from build123d import *

# Parameters (mm, degrees)
F1_DEPTH = 240
F0_W     = 160
F0_H     = 48
F0_W_2   = 40
F0_W_3   = 152
F0_H_2   = 202
F0_W_4   = 50
F0_H_3   = 150
F0_H_4   = 50
F2_DEPTH = 3
F3_DEPTH = 201
F4_DEPTH = 55
F5_DEPTH = 60
F6_DEPTH = 78


with BuildPart() as f1:
    # F0 (on Top) → F1 (new body)
    with BuildSketch(Plane.XY):
        Polygon((145, -391.5), (145, -373), (208, -373), (208, -391.5), (399.5, -391.5), (399.5, -68.5), (91, -68.5), (91, 10), (-10, 10), (-10, -391.5), align=None)
        Polygon((0, -381.5), (0, 0), (81, 0), (81, -78.5), (389.5, -78.5), (389.5, -381.5), (218, -381.5), (218, -363), (135, -363), (135, -381.5), align=None, mode=Mode.SUBTRACT)
    extrude(amount=F1_DEPTH)

    # F0 (on Top) → F2 (join)
    with BuildSketch(Plane.XY):
        Polygon((145, -391.5), (145, -373), (208, -373), (208, -391.5), (399.5, -391.5), (399.5, -68.5), (91, -68.5), (91, 10), (-10, 10), (-10, -391.5), align=None)
        Polygon((0, -381.5), (0, 0), (81, 0), (81, -78.5), (389.5, -78.5), (389.5, -381.5), (218, -381.5), (218, -363), (135, -363), (135, -381.5), align=None, mode=Mode.SUBTRACT)
        Polygon((81, 0), (0, 0), (0, -381.5), (135, -381.5), (135, -363), (218, -363), (218, -381.5), (389.5, -381.5), (389.5, -78.5), (81, -78.5), align=None)
        Polygon((2, -306.5), (2, -156.5), (52, -156.5), (52, -306.5), (75, -329.5), (125, -329.5), (125, -379.5), (75, -379.5), (2, -379.5), align=None, mode=Mode.SUBTRACT)
        with Locations((304.5, -355.5)):
            Rectangle(F0_W, F0_H, mode=Mode.SUBTRACT)
        with Locations((123.5, -107.5)):
            Rectangle(F0_W_2, F0_H, mode=Mode.SUBTRACT)
        with Locations((224.5, -184.5)):
            Rectangle(F0_W_3, F0_H_2, mode=Mode.SUBTRACT)
        with Locations((325.5, -107.5)):
            Rectangle(F0_W_2, F0_H, mode=Mode.SUBTRACT)
        with Locations((27, -231.5)):
            Rectangle(F0_W_4, F0_H_3)
        with Locations((224.5, -184.5)):
            Rectangle(F0_W_3, F0_H_2)
        with Locations((123.5, -107.5)):
            Rectangle(F0_W_2, F0_H)
        with Locations((325.5, -107.5)):
            Rectangle(F0_W_2, F0_H)
        with Locations((304.5, -355.5)):
            Rectangle(F0_W, F0_H)
        Polygon((52, -306.5), (2, -306.5), (2, -379.5), (75, -379.5), (75, -329.5), align=None)
        with Locations((100, -354.5)):
            Rectangle(F0_W_4, F0_H_4)
    extrude(amount=-F2_DEPTH)

    # F0 (on Top) → F3 (join)
    with BuildSketch(Plane.XY):
        with Locations((27, -231.5)):
            Rectangle(F0_W_4, F0_H_3)
        Polygon((52, -306.5), (2, -306.5), (2, -379.5), (75, -379.5), (75, -329.5), align=None)
        with Locations((100, -354.5)):
            Rectangle(F0_W_4, F0_H_4)
    extrude(amount=F3_DEPTH)

    # F0 (on Top) → F4 (join)
    with BuildSketch(Plane.XY):
        with Locations((123.5, -107.5)):
            Rectangle(F0_W_2, F0_H)
        with Locations((325.5, -107.5)):
            Rectangle(F0_W_2, F0_H)
    extrude(amount=F4_DEPTH)

    # F0 (on Top) → F5 (join)
    with BuildSketch(Plane.XY):
        with Locations((224.5, -184.5)):
            Rectangle(F0_W_3, F0_H_2)
    extrude(amount=F5_DEPTH)

    # F0 (on Top) → F6 (join)
    with BuildSketch(Plane.XY):
        with Locations((304.5, -355.5)):
            Rectangle(F0_W, F0_H)
    extrude(amount=F6_DEPTH)


solid = f1.part
The model under review builds one solid part; all positions refer to its coordinate system, in mm. A direction names the side the tool comes from. Give positions to 0.01 mm unless a question says otherwise; leave off trailing zeros. Order: outer loops, then holes, each group sorted by start corner. A loop starts at its lowest first (then second) coordinate and runs counter-clockwise, first axis right, second up. Notation, with made-up numbers: (69.25, 30) -> (105.25, 30) arc R16 ccw to (105.25, 45) -> close; hole circle Ø10 at (78, 8). An arc over 180 degrees is marked (long way). Write item = value, one per line. Start each with the question number.
(1) For pin 1 Ø20 at (x, y) = (132, -114.5) entering from +Z; pin 2 Ø12 at (x, y) = (37, -60.5) entering from +Z; pin 3 Ø1.5 at (x, y) = (48, -185.5) entering from +Z, all flat-tipped, find the tip position at first contact; note any pin that passes through.
(2) Take a section at A-A (z = 146). Write out the cut boundary in (x, y).
(3) Tool access review of faces 5 (the flat face through (52, -233, 99)), 6 (the flat face through (247, -68.5, 120)), 7 (the flat face through (176, -373, 120)): name each direction out of +Z, -Z, +X, -X, +Y, -Y from which nothing blocks a thin tool from reaching the whole face with its end or side.
(4) Take a section at C-C (y = -226). Write out the cut boundary in (x, z).
(5) Take a section at D-D (x = 157). Write out the cut boundary in (y, z), plus the area to 3 significant figures.
(6) Take a section at B-B (z = 224.5). Write out the cut boundary in (x, y).
(7) For L1, parallel to Y at x = 333, z = 54; L2, parallel to Y at x = 281.5, z = 38; L3, parallel to X at y = -365, z = 199, list the stretches that pass through material, from the lowest coordinate up. Write a range as from..to.
(8) Draft analysis for pull direction X (two halves, no side actions). For faces 1 (the flat face through (223, -83.5, 30)), 2 (the flat face through (302, -391.5, 120)), 3 (the flat face through (0, -193, 118)), 4 (the flat face through (399.5, -232, 120)), state which applies: +X half, -X half, draft (parallel to the pull), parting line (faces both ways), or undercut.
Returned:
q1.pin_1 = 55
q1.pin_2 = 0
q1.pin_3 = 201
q2.outline = (-10, -391.5) -> (145, -391.5) -> (145, -373) -> (208, -373) -> (208, -391.5) -> (399.5, -391.5) -> (399.5, -68.5) -> (91, -68.5) -> (91, 10) -> (-10, 10) -> close; (2, -379.5) -> (125, -379.5) -> (125, -329.5) -> (75, -329.5) -> (52, -306.5) -> (52, -156.5) -> (2, -156.5) -> close; hole (0, -381.5) -> (135, -381.5) -> (135, -363) -> (218, -363) -> (218, -381.5) -> (389.5, -381.5) -> (389.5, -78.5) -> (81, -78.5) -> (81, 0) -> (0, 0) -> close
q3.face_5 = +Z
q3.face_6 = +Z, -Z, +X, +Y
q3.face_7 = +Z, -Z, -Y
q4.outline = (-10, -3) -> (399.5, -3) -> (399.5, 240) -> (389.5, 240) -> (389.5, 0) -> (300.5, 0) -> (300.5, 60) -> (148.5, 60) -> (148.5, 0) -> (52, 0) -> (52, 201) -> (2, 201) -> (2, 0) -> (0, 0) -> (0, 240) -> (-10, 240) -> close
q5.outline = (-373, -3) -> (-68.5, -3) -> (-68.5, 240) -> (-78.5, 240) -> (-78.5, 0) -> (-83.5, 0) -> (-83.5, 60) -> (-285.5, 60) -> (-285.5, 0) -> (-363, 0) -> (-363, 240) -> (-373, 240) -> close
q5.area = 17,800 mm²
q6.outline = (-10, -391.5) -> (145, -391.5) -> (145, -373) -> (208, -373) -> (208, -391.5) -> (399.5, -391.5) -> (399.5, -68.5) -> (91, -68.5) -> (91, 10) -> (-10, 10) -> close; hole (0, -381.5) -> (135, -381.5) -> (135, -363) -> (218, -363) -> (218, -381.5) -> (389.5, -381.5) -> (389.5, -78.5) -> (81, -78.5) -> (81, 0) -> (0, 0) -> close
q7.L1 = -391.5..-381.5, -379.5..-331.5, -131.5..-83.5, -78.5..-68.5
q7.L2 = -391.5..-381.5, -379.5..-331.5, -285.5..-83.5, -78.5..-68.5
q7.L3 = -10..0, 2..125, 135..218, 389.5..399.5
q8.face_1 = undercut
q8.face_2 = draft
q8.face_3 = undercut
q8.face_4 = +X half
